For this review, take the finished solid that the model builds, in its own axes (mm). Coordinates: 2 decimals unless noted, no trailing zeros. Loops run counter-clockwise (first coordinate to the right, second up) from the corner with the lowest first, then second, coordinate; pieces in that order, holes last. Notation, with made-up numbers: M 41,54.25 L 45,54.25 A20 cw 45,58.25 Z; hole C -2.5,-27 d8. An arc over 180 degrees is marked long. Put each result on its own line as item: value.
Autodesk Inventor part; units mm, degrees
ref_plane "YZ Plane" through (0, 0, 0) normal (1, 0, 0) x (0, 1, 0)
ref_plane "XZ Plane" through (0, 0, 0) normal (0, 1, 0) x (-1, 0, 0)
ref_plane "XY Plane" through (0, 0, 0) normal (0, 0, 1) x (1, 0, 0)
sketch "Esquisse1" plane through (0, 0, 0) normal (0, 1, 0) x (-1, 0, 0)
  line L0 (81.9588, 98.0854) -> (-168.0412, 98.0854)
  line L1 (-168.0412, 98.0854) -> (-168.0412, -201.9146)
  line L2 (-168.0412, -201.9146) -> (81.9588, -201.9146)
  line L3 (81.9588, -201.9146) -> (81.9588, 98.0854)
  point P0 (0, 0)
  dimension "d0" = 300
  dimension "d1" = 250
extrude "Extrusion1" add sketch "Esquisse1" along normal blind 5
sketch "Sketch3" plane through (0, 5, 0) normal (0, 1, 0) x (1, 0, 0)
  line L0 (81.0412, -85.0854) -> (5.0412, -85.0854)
  line L1 (5.0412, -85.0854) -> (5.0412, -17.0854)
  line L2 (81.0412, -17.0854) -> (81.0412, -85.0854)
  line L3 (-81.9588, -98.0854) -> (168.0412, -98.0854)
  line L4 (168.0412, -98.0854) -> (168.0412, 201.9146)
  line L5 (17.0412, -17.0854) -> (17.0412, 40.9146)
  line L6 (17.0412, 40.9146) -> (69.0412, 40.9146)
  line L7 (69.0412, 40.9146) -> (69.0412, -17.0854)
  line L8 (5.0412, -17.0854) -> (17.0412, -17.0854)
  line L9 (69.0412, -17.0854) -> (81.0412, -17.0854)
  line L10 (81.0412, 188.9146) -> (5.0412, 188.9146)
  line L11 (5.0412, 188.9146) -> (5.0412, 120.9146)
  line L12 (81.0412, 120.9146) -> (81.0412, 188.9146)
  line L13 (168.0412, 201.9146) -> (-81.9588, 201.9146)
  line L14 (17.0412, 120.9146) -> (17.0412, 62.9146)
  line L15 (17.0412, 62.9146) -> (69.0412, 62.9146)
  line L16 (69.0412, 62.9146) -> (69.0412, 120.9146)
  line L17 (5.0412, 120.9146) -> (17.0412, 120.9146)
  line L18 (69.0412, 120.9146) -> (81.0412, 120.9146)
  circle A0 centre (85.0412, 51.9146) radius 1.5
  line L19 (-81.9588, 201.9146) -> (-81.9588, -98.0854)
  circle A1 centre (1.0412, 51.9146) radius 1.5
  point P0 (0, 0)
  dimension "d17" = 76
  dimension "d18" = 68
  dimension "d19" = 13
  dimension "d20" = 87
  dimension "d21" = 12
  dimension "d22" = 12
  dimension "d23" = 58
  dimension "d24" = 68
  dimension "d25" = 52
  dimension "d26" = 13
  dimension "d27" = 76
  dimension "d28" = 68
  dimension "d29" = 87
  dimension "d30" = 12
  dimension "d31" = 12
  dimension "d32" = 58
  dimension "d33" = 52
  dimension "d34" = 68
  dimension "d39" = 3
  dimension "d53" = 83
  dimension "d54" = 150
  dimension "d58" = 3
  dimension "d59" = 83
  dimension "d60" = 150
extrude "Extrusion3" cut sketch "Sketch3" against normal through all contours L0 L1 L8 L5 L6 L7 L9 L2 | L12 L18 L16 L15 L14 L17 L11 L10 | A0 | A1
sketch "Sketch4" plane through (0, 5, 0) normal (0, 1, 0) x (1, 0, 0)
  circle A0 centre (1.0412, -89.0854) radius 1.5
  circle A1 centre (1.0412, -11.0854) radius 1.5
  circle A2 centre (85.0412, -89.0854) radius 1.5
  circle A3 centre (85.0412, -11.0854) radius 1.5
  circle A4 centre (1.0412, 114.9146) radius 1.5
  circle A5 centre (1.0412, 192.9146) radius 1.5
  circle A6 centre (85.0412, 192.9146) radius 1.5
  circle A7 centre (85.0412, 114.9146) radius 1.5
  point P0 (0, 0)
extrude "Extrusion4" cut sketch "Sketch4" against normal up to next
sketch "Esquisse5" plane through (0, 5, 0) normal (0, 1, 0) x (1, 0, 0)
  circle A0 centre (139.5412, -83.0854) radius 1.5
  circle A1 centre (133.0412, -83.0854) radius 1.5
  circle A2 centre (133.0412, 186.9146) radius 1.5
  circle A3 centre (139.5412, 186.9146) radius 1.5
  circle A4 centre (-41.9588, 186.9146) radius 1.5
  circle A5 centre (-48.4588, 186.9145) radius 1.4999
  circle A6 centre (-41.9588, -83.0854) radius 1.5
  circle A7 centre (85.0412, 192.9146) radius 1.5
  circle A8 centre (1.0412, 114.9146) radius 1.5
  circle A9 centre (85.0412, -89.0854) radius 1.5
  circle A10 centre (1.0412, -89.0854) radius 1.5
  circle A11 centre (1.0412, -11.0854) radius 1.5
  circle A12 centre (85.0412, -11.0854) radius 1.5
  circle A13 centre (1.0412, 192.9146) radius 1.5
  circle A14 centre (85.0412, 114.9146) radius 1.5
  line L0 (81.0412, -17.0854) -> (81.0412, -85.0854)
  line L1 (81.0412, -85.0854) -> (5.0412, -85.0854)
  line L2 (5.0412, -85.0854) -> (5.0412, -17.0854)
  line L3 (5.0412, -17.0854) -> (17.0412, -17.0854)
  line L4 (17.0412, -17.0854) -> (17.0412, 40.9146)
  line L5 (17.0412, 40.9146) -> (69.0412, 40.9146)
  line L6 (69.0412, 40.9146) -> (69.0412, -17.0854)
  line L7 (69.0412, -17.0854) -> (81.0412, -17.0854)
  circle A15 centre (85.0412, 51.9146) radius 1.5
  circle A16 centre (1.0412, 51.9146) radius 1.5
  line L8 (5.0412, 120.9146) -> (5.0412, 188.9146)
  line L9 (5.0412, 188.9146) -> (81.0412, 188.9146)
  line L10 (81.0412, 188.9146) -> (81.0412, 120.9146)
  line L11 (81.0412, 120.9146) -> (69.0412, 120.9146)
  line L12 (69.0412, 120.9146) -> (69.0412, 62.9146)
  line L13 (69.0412, 62.9146) -> (17.0412, 62.9146)
  line L14 (17.0412, 62.9146) -> (17.0412, 120.9146)
  line L15 (17.0412, 120.9146) -> (5.0412, 120.9146)
  line L16 (-81.9588, -98.0854) -> (168.0412, -98.0854)
  line L17 (168.0412, -98.0854) -> (168.0412, 201.9146)
  line L18 (168.0412, 201.9146) -> (-81.9588, 201.9146)
  line L19 (-81.9588, 201.9146) -> (-81.9588, -98.0854)
  circle A17 centre (-48.4588, -83.0854) radius 1.5
  point P0 (0, 0)
extrude "Extrusion5" cut sketch "Esquisse5" against normal up to next contours A0 | A1 | A2 | A3 | A4 | A5 | A6 | A17
sketch "Esquisse6" plane through (0, 0, 0) normal (0, -1, 0) x (1, 0, 0)
  circle A0 centre (-76.9588, -142.9146) radius 1.5
  circle A1 centre (-52.9588, -166.9146) radius 1.5
  circle A2 centre (-76.9588, 63.0854) radius 1.5
  circle A3 centre (-52.9588, 39.0854) radius 1.5
  circle A4 centre (139.0412, 63.0854) radius 1.5
  circle A5 centre (163.0412, 39.0854) radius 1.5
  circle A6 centre (139.0412, -142.9146) radius 1.5
  circle A7 centre (163.0412, -166.9146) radius 1.5
  point P0 (0, 0)
extrude "Extrusion6" cut sketch "Esquisse6" against normal up to next
sketch "Esquisse7" plane through (0, 5, 0) normal (0, 1, 0) x (1, 0, 0)
  circle A0 centre (152.0412, 161.9146) radius 1.5
  circle A1 centre (-65.9588, 51.9146) radius 1.5
  circle A2 centre (152.0412, 51.9146) radius 1.5
  circle A3 centre (152.0412, -58.0854) radius 1.5
  line L0 (-81.9588, 201.9146) -> (168.0412, 201.9146)
  line L1 (-81.9588, -98.0854) -> (-81.9588, 201.9146)
  line L2 (168.0412, -98.0854) -> (-81.9588, -98.0854)
  line L3 (168.0412, 201.9146) -> (168.0412, -98.0854)
  circle A4 centre (152.0412, 161.9146) radius 1.5
  circle A5 centre (-65.9588, 51.9146) radius 1.5
  circle A6 centre (152.0412, 51.9146) radius 1.5
  circle A7 centre (152.0412, -58.0854) radius 1.5
  line L4 (-81.9588, 201.9146) -> (168.0412, 201.9146)
  line L5 (-81.9588, -98.0854) -> (-81.9588, 201.9146)
  line L6 (168.0412, -98.0854) -> (-81.9588, -98.0854)
  line L7 (168.0412, 201.9146) -> (168.0412, -98.0854)
  circle A8 centre (152.0412, 161.9146) radius 1.5
  circle A9 centre (-65.9588, 51.9146) radius 1.5
  circle A10 centre (152.0412, 51.9146) radius 1.5
  circle A11 centre (152.0412, -58.0854) radius 1.5
  line L8 (-81.9588, 201.9146) -> (168.0412, 201.9146)
  line L9 (-81.9588, -98.0854) -> (-81.9588, 201.9146)
  line L10 (168.0412, -98.0854) -> (-81.9588, -98.0854)
  line L11 (168.0412, 201.9146) -> (168.0412, -98.0854)
  circle A12 centre (139.0412, 142.9146) radius 1.5
  circle A13 centre (139.0412, -63.0854) radius 1.5
  circle A14 centre (-76.9588, -63.0854) radius 1.5
  circle A15 centre (-76.9588, 142.9146) radius 1.5
  circle A16 centre (-52.9588, 166.9146) radius 1.5
  circle A17 centre (-52.9588, -39.0854) radius 1.5
  circle A18 centre (163.0412, -39.0854) radius 1.5
  circle A19 centre (163.0412, 166.9146) radius 1.5
  circle A20 centre (133.0412, -83.0854) radius 1.5
  circle A21 centre (-41.9588, 186.9146) radius 1.5
  circle A22 centre (133.0412, 186.9146) radius 1.5
  circle A23 centre (-48.4588, 186.9145) radius 1.4999
  circle A24 centre (139.5412, 186.9146) radius 1.5
  circle A25 centre (-41.9588, -83.0854) radius 1.5
  circle A26 centre (139.5412, -83.0854) radius 1.5
  circle A27 centre (-48.4588, -83.0854) radius 1.5
  circle A28 centre (85.0412, 192.9146) radius 1.5
  circle A29 centre (1.0412, 114.9146) radius 1.5
  circle A30 centre (85.0412, -89.0854) radius 1.5
  circle A31 centre (1.0412, -89.0854) radius 1.5
  circle A32 centre (1.0412, -11.0854) radius 1.5
  circle A33 centre (85.0412, -11.0854) radius 1.5
  circle A34 centre (1.0412, 192.9146) radius 1.5
  circle A35 centre (85.0412, 114.9146) radius 1.5
  line L12 (81.0412, -17.0854) -> (81.0412, -85.0854)
  line L13 (81.0412, -85.0854) -> (5.0412, -85.0854)
  line L14 (5.0412, -85.0854) -> (5.0412, -17.0854)
  line L15 (5.0412, -17.0854) -> (17.0412, -17.0854)
  line L16 (17.0412, -17.0854) -> (17.0412, 40.9146)
  line L17 (17.0412, 40.9146) -> (69.0412, 40.9146)
  line L18 (69.0412, 40.9146) -> (69.0412, -17.0854)
  line L19 (69.0412, -17.0854) -> (81.0412, -17.0854)
  circle A36 centre (85.0412, 51.9146) radius 1.5
  circle A37 centre (1.0412, 51.9146) radius 1.5
  line L20 (5.0412, 120.9146) -> (5.0412, 188.9146)
  line L21 (5.0412, 188.9146) -> (81.0412, 188.9146)
  line L22 (81.0412, 188.9146) -> (81.0412, 120.9146)
  line L23 (81.0412, 120.9146) -> (69.0412, 120.9146)
  line L24 (69.0412, 120.9146) -> (69.0412, 62.9146)
  line L25 (69.0412, 62.9146) -> (17.0412, 62.9146)
  line L26 (17.0412, 62.9146) -> (17.0412, 120.9146)
  line L27 (17.0412, 120.9146) -> (5.0412, 120.9146)
  line L28 (-81.9588, -98.0854) -> (168.0412, -98.0854)
  line L29 (168.0412, -98.0854) -> (168.0412, 201.9146)
  line L30 (168.0412, 201.9146) -> (-81.9588, 201.9146)
  line L31 (-81.9588, 201.9146) -> (-81.9588, -98.0854)
  circle A38 centre (100.5413, 149.4146) radius 2.0001
  circle A39 centre (120.5412, 149.4146) radius 2
  circle A40 centre (100.5412, -45.5854) radius 2
  circle A41 centre (120.5412, -45.5854) radius 2
  circle A42 centre (75.0412, 19.9146) radius 2
  circle A43 centre (11.0412, 83.9146) radius 2
  circle A44 centre (11.0412, 19.9146) radius 2
  circle A45 centre (75.0412, 83.9146) radius 2
  circle A46 centre (-61.9588, 171.9146) radius 7.5
  circle A47 centre (75.0412, 19.9146) radius 2
  circle A48 centre (11.0412, 83.9146) radius 2
  circle A49 centre (11.0412, 19.9146) radius 2
  circle A50 centre (75.0412, 83.9146) radius 2
  circle A51 centre (-61.9588, 171.9146) radius 7.5
  circle A52 centre (75.0412, 19.9146) radius 2
  circle A53 centre (11.0412, 83.9146) radius 2
  circle A54 centre (11.0412, 19.9146) radius 2
  circle A55 centre (75.0412, 83.9146) radius 2
  circle A56 centre (-61.9588, 171.9146) radius 7.5
  point P0 (0, 0)
extrude "Extrusion7" cut sketch "Esquisse7" against normal up to next contours A38 | A39 | A40 | A41
properties part number "socle-robot"
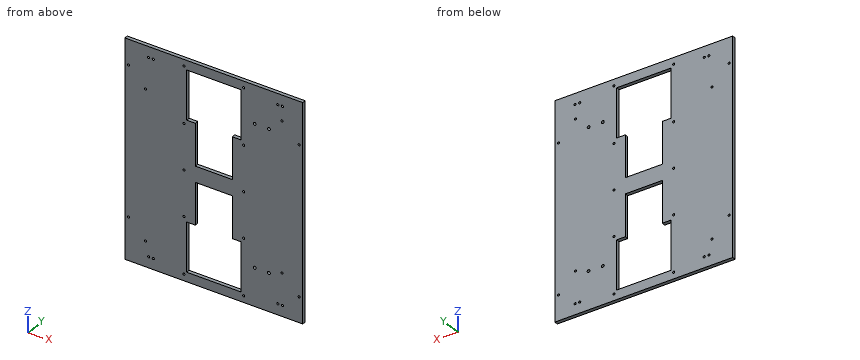
(1) Add section B-B (x = 12). Write out the cut boundary in (y, z).
Determined:
outline: M 0,-201.91 L 5,-201.91 L 5,-188.91 L 0,-188.91 Z; M 0,-120.91 L 5,-120.91 L 5,17.09 L 0,17.09 Z; M 0,85.09 L 5,85.09 L 5,98.09 L 0,98.09 Z
(2) Add section D-D (x = 48). Write out the cut boundary in (y, z), plus the area to 3 significant figures.
Determined:
outline: M 0,-201.91 L 5,-201.91 L 5,-188.91 L 0,-188.91 Z; M 0,-62.91 L 5,-62.91 L 5,-40.91 L 0,-40.91 Z; M 0,85.09 L 5,85.09 L 5,98.09 L 0,98.09 Z
area: 240 mm^2
(3) Add section C-C (z = -5). Write out the cut boundary in (x, y), plus the area to 3 significant figures.
Determined:
outline: M -81.96,0 L 17.04,0 L 17.04,5 L -81.96,5 Z; M 69.04,0 L 168.04,0 L 168.04,5 L 69.04,5 Z
area: 990 mm^2
(4) Add section A-A (z = 78). Write out the cut boundary in (x, y).
Determined:
outline: M -81.96,0 L 5.04,0 L 5.04,5 L -81.96,5 Z; M 81.04,0 L 168.04,0 L 168.04,5 L 81.04,5 Z
(5) Wall thickness on line 1 along Z through (x, y) = (12, 0.25); line 2 along Z through (x, y) = (34.5, 4.25); line 3 along X through (y, z) = (3.9, 72): over which ranges is each line inside the solid? List them lowest first. Write a range as [from, to].
Determined:
line 1: z = [-201.91, -188.91], [-120.91, 17.09], [85.09, 98.09]
line 2: z = [-201.91, -188.91], [-62.91, -40.91], [85.09, 98.09]
line 3: x = [-81.96, 5.04], [81.04, 168.04]
